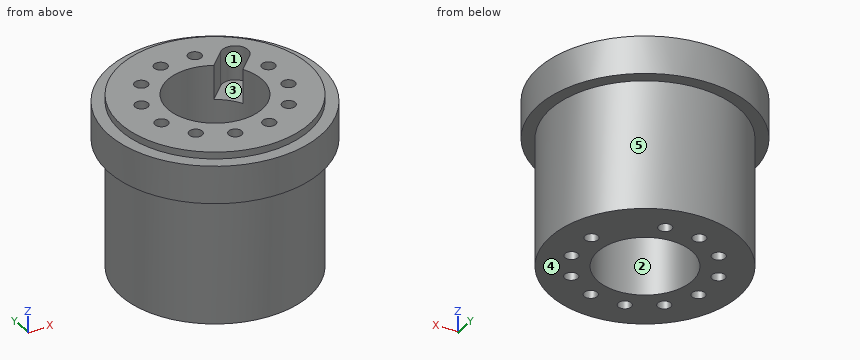
from build123d import *

# Parameters (mm, degrees)
SKETCH_1_R               = 6.2
SKETCH_1_R_2             = 2.75
EXTRUDE_1_DEPTH          = 2.2
SKETCH_1_5_R             = 5.5
SKETCH_1_5_R_2           = 2.75
EXTRUDE_3_DEPTH          = 7.5
EXTRUDE_START            = 2.2
SKETCH_1_6_R             = 5.5
SKETCH_1_6_R_2           = 2.75
EXTRUDE_4_DEPTH          = 0.4
SKETCH_2_R               = 0.381
CUT_EXTRUDE_1_DEPTH      = 14.374976635
PATTERN_CIRCULAR_1_COUNT = 12
CUT_EXTRUDE_2_DEPTH      = 2


with BuildPart() as part:
    # Sketch 1 → Extrude 1 (new body)
    with BuildSketch(Plane.XY):
        Circle(SKETCH_1_R)
        Circle(SKETCH_1_R_2, mode=Mode.SUBTRACT)
    extrude(amount=EXTRUDE_1_DEPTH)

    # Sketch 1_5 → Extrude 3 (add)
    with BuildSketch(Plane.XY):
        Circle(SKETCH_1_5_R)
        Circle(SKETCH_1_5_R_2, mode=Mode.SUBTRACT)
    extrude(amount=-EXTRUDE_3_DEPTH)

    # Sketch 1_6 → Extrude 4 (add)
    with BuildSketch(Plane.XY.offset(EXTRUDE_START)):
        Circle(SKETCH_1_6_R)
        Circle(SKETCH_1_6_R_2, mode=Mode.SUBTRACT)
    extrude(amount=EXTRUDE_4_DEPTH)

    # Sketch 2 → Cut-Extrude 1 (cut, through all)
    with BuildSketch(Plane.XY.offset(2.6)):
        with Locations((0.986100562, 3.680177398)):
            Circle(SKETCH_2_R)
    cut_extrude_1 = extrude(amount=-CUT_EXTRUDE_1_DEPTH, mode=Mode.SUBTRACT)

    # Pattern Circular 1: Cut-Extrude 1 ×12 about axis, 1 skipped
    pattern_circular_1_axis = Axis((0, 0, 0), (0, 0, 1))
    add([cut_extrude_1.rotate(pattern_circular_1_axis, i * 360 / PATTERN_CIRCULAR_1_COUNT) for i in range(1, PATTERN_CIRCULAR_1_COUNT) if i not in (11,)], mode=Mode.SUBTRACT)

    # Sketch 4 → Cut-Extrude 2 (cut)
    with BuildSketch(Plane.XY.offset(2.6)):
        with BuildLine():
            ThreePointArc((1.340498607, 2.401158779), (1.944543648, 1.944543648), (2.401158779, 1.340498607))
            Line((2.401158779, 1.340498607), (3.358757211, 2.298097039))
            ThreePointArc((3.358757211, 2.298097039), (3.358757211, 3.358757211), (2.298097039, 3.358757211))
            Line((2.298097039, 3.358757211), (1.340498607, 2.401158779))
        make_face()
    extrude(amount=-CUT_EXTRUDE_2_DEPTH, mode=Mode.SUBTRACT)


solid = part.part
Part model, mm, in its own coordinate system. Face numbers are marked on the shaded views. A direction names the side the tool comes from. Give positions to 0.01 mm unless a question says otherwise; leave off trailing zeros. Order: outer loops, then holes, each group sorted by start corner. A loop starts at its lowest first (then second) coordinate and runs counter-clockwise, first axis right, second up. Notation, with made-up numbers: (33.5, 22) - (68.5, 22) arc R12 ccw to (68.5, 26) - close; hole circle Ø9 at (23, 88). An arc over 180 degrees is marked (long way). One line per question, with ' | ' between items.
1. Band-saw the part on C-C on z = 0.25. Give the number of separate pieces and of enclosed holes in the cut face, then the cut area to 3 significant figures.
Filled in:
separate pieces: 1 | enclosed holes: 12 | area: 92.0 mm²
2. Drop flat-ended pins along their axis: P1, Ø6, axis at x = 2, z = -2.5, coming from the +Y side; P2, Ø1.5, axis at x = 0, z = -6, coming from the +Y side; P3, Ø2, axis at y = -2.5, z = 0.5, coming from the -X side. Give the stop position or say it passes through.
Filled in:
P1: y = 6.19 | P2: y = 5.5 | P3: x = -6.02
3. Band-saw the part on D-D on y = -5. List the corners of the cut face in (x, z).
Filled in:
outline: (-3.67, 0) - (-2.29, 0) - (-2.29, -7.5) - (2.29, -7.5) - (2.29, 0) - (3.67, 0) - (3.67, 2.2) - (2.29, 2.2) - (2.29, 2.6) - (-2.29, 2.6) - (-2.29, 2.2) - (-3.67, 2.2) - close
4. Drill centre lines: probe 1 along X at (y, z) = (-2.5, -0.5); probe 2 along Y at (x, z) = (-4, -0.5); probe 3 along Y at (x, z) = (-1.25, -4.5). Where is each one in solid material? Low to high.
Filled in:
probe 1: -4.9 to -3.02, -2.37 to -1.15, 1.15 to 2.37, 3.02 to 4.9 | probe 2: -3.77 to -1.19, -0.78 to 0.78, 1.19 to 3.77 | probe 3: -5.36 to -3.95, -3.41 to -2.45, 2.45 to 3.41, 3.95 to 5.36
5. Band-saw the part on A-A on y = 0. List the corners of the cut face in (x, z).
Filled in:
outline: (-6.2, 0) - (-5.5, 0) - (-5.5, -7.5) - (-2.75, -7.5) - (-2.75, 2.6) - (-5.5, 2.6) - (-5.5, 2.2) - (-6.2, 2.2) - close; (2.75, -7.5) - (5.5, -7.5) - (5.5, 0) - (6.2, 0) - (6.2, 2.2) - (5.5, 2.2) - (5.5, 2.6) - (2.75, 2.6) - close
6. Pull direction Y, two halves, no side cores. Call the marked faces 3, 4 and 5: +Y half, -Y half, draft (parallel to the pull), parting line (faces both ways), or undercut.
Filled in:
face 3: undercut | face 4: draft | face 5: parting line
7. Which spindle directions (+Z, -Z, +X, -X, +Y, -Y) get a long thin tool onto all of the face, cutting with end or side? Do the marked faces 1 and 2. Say none if no direction does.
Filled in:
face 1: +Z | face 2: +Z, -Z
